Part model, mm, in its own coordinate system. Coordinates: 2 decimals unless noted, no trailing zeros. Write each loop counter-clockwise with the first axis right and the second up, starting at its lowest first coordinate (ties: lowest second). Pieces come first, ordered by that corner, then holes. Notation, with made-up numbers: (24, 70.25) -> (58, 70.25) arc R27 ccw to (58, 107.25) -> close; hole circle Ø8 at (85.25, 46.25). An arc over 180 degrees is marked (long way). One line per question, with ' | ' between items. Start each with the question number.
Item 1: Probe probe 1 along Z at (x, y) = (-2.85, 22); probe 2 along Z at (x, y) = (-1.2, 3.5). List the from-to ranges inside material, lowest first. Write a range as [from, to].
Item 2: Saw through at A-A (x = -0.95). List the corners of the cut face in (y, z) (3 decimals), and give its area (3 significant figures).
Item 3: Pin check, flat tip, straight feed: pin 1 (1 mm diameter, centred on x = -1, y = 43.5, fed in from -Z). Stop position of the tip, or through.
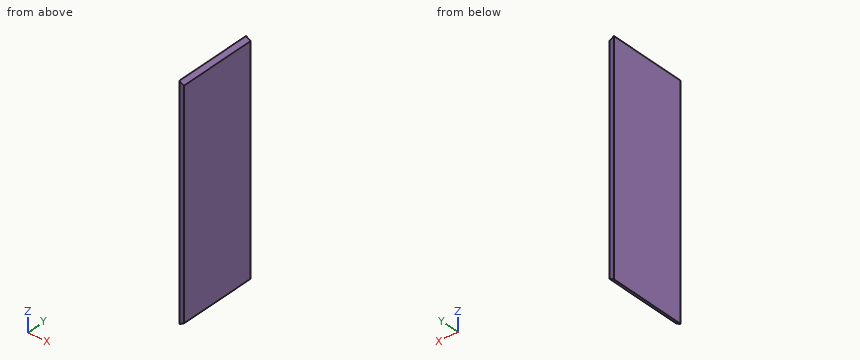
Autodesk Inventor part; units mm, degrees
ref_plane "Work Plane1" through (0, 0, -76.2) normal (0, 0, -1) x (-1, 0, 0)
ref_plane "YZ Plane" through (0, 0, 0) normal (1, 0, 0) x (0, 1, 0)
ref_plane "XZ Plane" through (0, 0, 0) normal (0, 1, 0) x (-1, 0, 0)
sketch "Sketch1" plane through (0, 0, 0) normal (0, 1, 0) x (-1, 0, 0)
  line L0 (0, 0) -> (3.175, 0)
  line L1 (3.175, 0) -> (3.175, -152.4)
  line L2 (3.175, -152.4) -> (0, -152.4)
  line L3 (0, -152.4) -> (0, 0)
  dimension "d0" = 3.175
  dimension "d1" = 152.4
extrude "Extrusion1" add sketch "Sketch1" along normal blind 53.975
sketch "Sketch2" plane through (0, 53.975, 0) normal (0, 1, 0) x (1, 0, 0)
  line L0 (-3.175, 152.4) -> (-3.175, 0)
  line L1 (-3.175, 0) -> (78.8226, -52.7127)
  line L2 (78.8226, -52.7127) -> (78.8226, -16.7976)
  line L3 (-3.175, 0) -> (11.7687, 8.1586)
  line L4 (0, 0) -> (0, 152.4)
  line L5 (0, 1.7334) -> (0, 0)
  line L6 (0, 0) -> (-3.175, 0)
  dimension "d4" = 57.265
  dimension "d5" = 61.368
ref_plane "Work Plane1" through (0, 0, -76.2) normal (0, 0, -1) x (-1, 0, 0)
extrude "Extrusion2" cut sketch "Sketch2" against normal blind 53.975
mirror "Mirror1" about plane through (0, 0, -76.2) normal (0, 0, -1) of "Extrusion2"
sketch "Sketch3" plane through (-3.175, 0, 0) normal (-1, 0, 0) x (0, 0, 1)
  line L0 (-152.4, 53.975) -> (0, 53.975)
  line L1 (-152.4, 0) -> (-152.4, 53.975)
  point P0 (0, 0)
  point P1 (-120.65, 44.45)
  point P2 (-31.75, 44.45)
  dimension "d8" = 9.525
  dimension "d9" = 31.75
  dimension "d10" = 31.75
properties part number "Back Wall"
From the geometry:
1) probe 1: [-152.22, -0.18] | probe 2: [-151.32, -1.08]
2) outline: (0, -151.185) -> (53.975, -151.185) -> (53.975, -1.215) -> (0, -1.215) -> close | area: 8,090 mm2
3) pin 1: z = -151.49
